Read the model definition and answer for the solid it produces. Units are mm, in the model's axes. A direction names the side the tool comes from. Give positions to 0.01 mm unless a question says otherwise; leave off trailing zeros. Order: outer loops, then holes, each group sorted by start corner. A loop starts at its lowest first (then second) coordinate and runs counter-clockwise, first axis right, second up.
Item 1: A cutting plane is placed at A-A (y = -6). Write down the section's boundary in (x, z).
Item 2: The mould has two halves that part along Z. Classify faces 3 (the face through (-3, 40, 0)), 4 (the face through (0.13, 21.68, 0.41)), 5 (the face through (1.38, 1.05, -6.2)): +Z half, -Z half, draft (parallel to the pull), parting line (faces both ways), or undercut.
Item 3: Given pin 1 Ø2 at (x, y) = (3.5, -25.5) entering from -Z; pin 2 Ø1 at (y, z) = (-14, -3) entering from -X; pin 3 Ø3 at (x, y) = (-5, -19) entering from +Z, each flat-ended and moving along its own axis, determine where each tip first touches the part or whether it passes through.
Item 4: Which of the six approach directions +Z, -Z, +X, -X, +Y, -Y give full straight-line access (tool end or side, diameter ignored) to faces 1 (the face through (0, -40, 0)), 2 (the face through (-0.738, 31.33, 2.345))?
Item 5: Find the intervals of material crossed by line 1 along Z through (x, y) = (0, 29); line 2 along X through (y, z) = (0, -5.25); line 3 along Y through (x, z) = (4.5, 3), in increasing order.
Autodesk Inventor part; units mm, degrees
ref_plane "YZ Plane" through (0, 0, 0) normal (1, 0, 0) x (0, 1, 0)
ref_plane "XZ Plane" through (0, 0, 0) normal (0, 1, 0) x (-1, 0, 0)
ref_plane "XY Plane" through (0, 0, 0) normal (0, 0, 1) x (1, 0, 0)
sketch "Sketch1" plane through (0, 0, 0) normal (0, 1, 0) x (-1, 0, 0)
  circle A0 centre (0, 0) radius 6.35
  dimension "d0" = 12.7
extrude "Extrusion1" add sketch "Sketch1" along normal mid plane 80
chamfer "Chamfer1" distance 1 angle 45 1 edges at (6.35, -40, 0)
hole "Hole3" at (0, 40, 0) direction (0, -1, 0) diameter 4.917 depth 17.1 tip angle 118
properties part number "suporte-barra" material "Aluminium AW-7020"
Response values:
1. outline: circle Ø12.7 at (0, 0)
2. face 3: draft
2. face 4: undercut
2. face 5: parting line
3. pin 1: stops at z = -5.84
3. pin 2: stops at x = -5.84
3. pin 3: stops at z = 5.3
4. face 1: +Z, -Z, +X, -X, -Y
4. face 2: +Y
5. line 1: z = -6.35 to -2.46, 2.46 to 6.35
5. line 2: x = -3.57 to 3.57
5. line 3: y = -39.94 to 40
